Design review of the part built by this model. Coordinates are the model's own, in mm. A direction names the side the tool comes from. Coordinates: 2 decimals unless noted, no trailing zeros. Loops run counter-clockwise (first coordinate to the right, second up) from the corner with the lowest first, then second, coordinate; pieces in that order, holes last. Notation, with made-up numbers: (71.25, -3.5) -> (110.25, -3.5) arc R22 ccw to (110.25, 13.5) -> close; hole circle Ø1 at (89.5, 45). An arc over 180 degrees is marked (long way). One line per item, written item: value. Start each with the question number.
1. For probe 1 along X at (y, z) = (31.5, -10.5); probe 2 along Y at (x, z) = (5, 13), list the stretches that pass through material, from the lowest coordinate up.
2. Add section A-A on z = -8. Write out the cut boundary in (x, y), plus the area to 3 significant figures.
3. Add section B-B on y = 4. Write out the cut boundary in (x, z), plus the area to 3 significant figures.
4. Insertion check: pin 1 (1.5 mm diameter, centred on x = 31.5, z = -1, fed in from +Y); pin 2 (8 mm diameter, centred on x = 16.5, z = -10.5, fed in from +Y); pin 3 (6 mm diameter, centred on y = 22, z = 9.5, fed in from +X). Each pin has a flat end and moves straight along its axis. Give the tip position at first contact, or say it passes through.
5. Machinability: for faces 1 (the flat face through (45, 10, 0)), 2 (the flat face through (5, 40, 0)), which of the approach directions +Z, -Z, +X, -X, +Y, -Y give a long, thin tool a straight path to every point of the face, cutting with its end or side? Answer none if there is none.
6. Add section C-C on x = 5. Write out the cut boundary in (y, z).
7. Add section D-D on z = -17. Write out the cut boundary in (x, y).
Autodesk Inventor part; units mm, degrees
ref_plane "YZ Plane" through (0, 0, 0) normal (1, 0, 0) x (0, 1, 0)
ref_plane "XZ Plane" through (0, 0, 0) normal (0, 1, 0) x (-1, 0, 0)
ref_plane "XY Plane" through (0, 0, 0) normal (0, 0, 1) x (1, 0, 0)
sketch "草圖1" plane through (0, 0, 0) normal (0, 1, 0) x (-1, 0, 0)
  line L0 (0, -20) -> (-60, -20)
  line L1 (-60, -20) -> (-60, 20)
  line L2 (-60, 20) -> (0, 20)
  line L3 (0, 20) -> (0, -20)
  point P0 (0, 0)
  point P1 (0, 0)
  dimension "d0" = 40
  dimension "d1" = 60
extrude "擠出1" add sketch "草圖1" along normal blind 40
sketch "草圖2" plane through (0, 0, 20) normal (0, 0, 1) x (1, 0, 0)
  line L0 (0, 0) -> (0, 40)
  line L1 (0, 40) -> (60, 40)
  line L2 (60, 40) -> (60, 0)
  line L3 (60, 0) -> (0, 0)
  line L4 (10, 40) -> (10, 20)
  line L5 (10, 20) -> (30, 10)
  line L6 (30, 10) -> (60, 10)
  line L7 (60, 0) -> (60, 40)
  dimension "d4" = 10
  dimension "d5" = 10
  dimension "d6" = 20
  dimension "d7" = 30
extrude "擠出2" cut sketch "草圖2" against normal through all contours L1 L2 L6 L5 L4
fillet "圓角1" radius 10 4 edges at (5, 40, 20) (5, 40, -20) (60, 5, 20) (60, 5, -20)
properties part number "33" material "鋼、碳鋼"
Worked answers:
1. probe 1: x = 0 to 10
1. probe 2: y = 0 to 39.54
2. outline: (0, 0) -> (60, 0) -> (60, 10) -> (30, 10) -> (10, 20) -> (10, 40) -> (0, 40) -> close
2. area: 1,000 mm²
3. outline: (0, -20) -> (50, -20) arc R10 ccw to (60, -10) -> (60, 10) arc R10 ccw to (50, 20) -> (0, 20) -> close
3. area: 2,360 mm²
4. pin 1: stops at y = 10
4. pin 2: stops at y = 18.75
4. pin 3: stops at x = 12
5. face 1: +Z, -Z, +X, +Y
5. face 2: +Z, -Z, +X, -X, +Y
6. outline: (0, -20) -> (30, -20) arc R10 ccw to (40, -10) -> (40, 10) arc R10 ccw to (30, 20) -> (0, 20) -> close
7. outline: (0, 0) -> (57.14, 0) -> (57.14, 10) -> (30, 10) -> (10, 20) -> (10, 37.14) -> (0, 37.14) -> close
